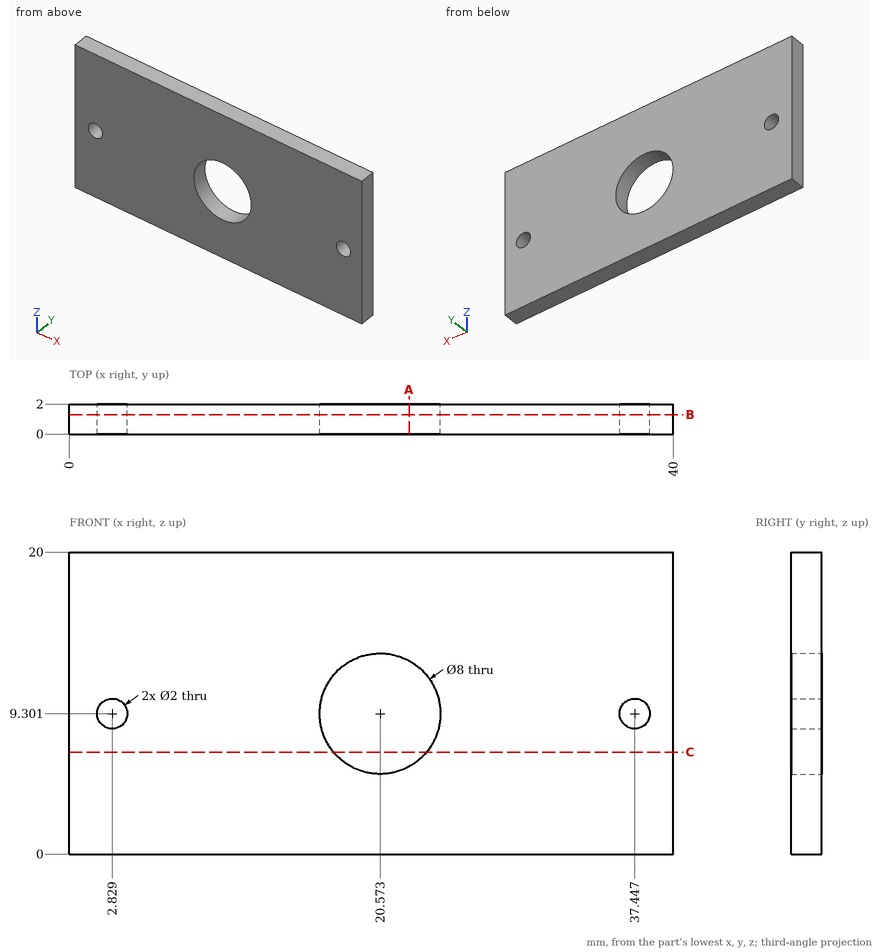
Could you check a few things on this drawing? It's one solid part, dimensions in mm from its lowest x, y, z. Give positions to 0.01 mm unless a question says otherwise; leave off trailing zeros. Loops run counter-clockwise (first coordinate to the right, second up) from the corner with the lowest first, then second, coordinate; pieces in that order, holes last. Notation, with made-up numbers: M 77,49.25 L 109,49.25 A18 ccw 109,60.25 Z; hole C 13.25,64 d1. An arc over 180 degrees is marked long. Return JSON: item names as keys, results as strings.
Item 1: Imagine slicing it at A-A on x = 22.5. List the corners of the cut face in (y, z) for me.
A:
{"outline": "M 0,0 L 2,0 L 2,5.8 L 0,5.8 Z; M 0,12.81 L 2,12.81 L 2,20 L 0,20 Z"}
Item 2: Imagine slicing it at C-C on z = 6.75. List the corners of the cut face in (x, y) for me.
A:
{"outline": "M 0,0 L 17.49,0 L 17.49,2 L 0,2 Z; M 23.65,0 L 40,0 L 40,2 L 23.65,2 Z"}
Item 3: Imagine slicing it at B-B on y = 1.3. List the corners of the cut face in (x, z) for me.
A:
{"outline": "M 0,0 L 40,0 L 40,20 L 0,20 Z; hole C 2.83,9.3 d2; hole C 20.57,9.3 d8; hole C 37.45,9.3 d2"}
Item 4: Please list where these lines run through material, in increasing order: line 1 (X direction, y = 1.7, z = 11) (1 decimal); line 2 (X direction, y = 1.85, z = 11.25); line 3 (Z direction, x = 23.5, y = 0.35) (1 decimal).
A:
{"line 1": "x = 0 to 17, 24.2 to 40", "line 2": "x = 0 to 17.08, 24.07 to 40", "line 3": "z = 0 to 6.6, 12 to 20"}
Item 5: I'm going to push flat-ended pins straight in: pin 1 Ø1.6 at (x, z) = (37.45, 9.3) entering from -Y; pin 2 Ø2.5 at (x, z) = (2.83, 9.3) entering from -Y. Where does each tip first touch, or does it pass through?
A:
{"pin 1": "passes through", "pin 2": "stops at y = 0"}
